from build123d import *

# Parameters (mm, degrees)
SKETCH1_R           = 35
BOSS_EXTRUDE1_DEPTH = 203.105968
SKETCH2_R           = 27.36149988
CUT_EXTRUDE1_DEPTH  = 210.050315085
CHAMFER1_SIZE       = 0.441228


with BuildPart() as part:
    # Sketch1 → Boss-Extrude1 (new body)
    with BuildSketch(Plane(origin=(0, 0, 0), x_dir=(1, 0, 0), z_dir=(0, 1, 0))):
        with Locations(Location((0, 0, 0), (0, 0, 270))):
            Circle(SKETCH1_R)
    extrude(amount=BOSS_EXTRUDE1_DEPTH)

    # Sketch2 → Cut-Extrude1 (cut, through all)
    with BuildSketch(Plane(origin=(0, 0, 0), x_dir=(1, 0, 0), z_dir=(0, 1, 0))):
        with Locations(Location((0, 0, 0), (0, 0, 270))):
            Circle(SKETCH2_R)
    extrude(amount=CUT_EXTRUDE1_DEPTH, mode=Mode.SUBTRACT)

    # Chamfer1
    chamfer1_edges = [part.edges().sort_by_distance(p)[0] for p in [
        (0, 0, -35),
        (0, 203.105968, -35),
        (0, 0, -27.36149988),
        (0, 203.105968, -27.36149988),
    ]]
    chamfer(chamfer1_edges, length=CHAMFER1_SIZE)


solid = part.part
Geometry: final body of the model. Coordinates: model frame, mm. Round coordinates to 2 decimals unless told otherwise and drop trailing zeros. Write each loop counter-clockwise with the first axis right and the second up, starting at its lowest first coordinate (ties: lowest second). Pieces come first, ordered by that corner, then holes. Notation, with made-up numbers: M 61.25,-11 L 95.25,-11 A16 ccw 95.25,4 Z; hole C -9.5,71.25 d8. An arc over 180 degrees is marked long. Write item = value, one per line.
Item 1: Section query C-C on y = 120.5. Return loops of the section in (x, z).
Findings:
outline = C 0,0 d70; hole C 0,0 d54.72
Item 2: Section query B-B on z = 0. Return loops of the section in (x, y), then the cut area to 3 significant figures.
Findings:
outline = M -35,0.44 L -34.56,0 L -27.8,0 L -27.36,0.44 L -27.36,202.66 L -27.8,203.11 L -34.56,203.11 L -35,202.66 Z; M 27.36,0.44 L 27.8,0 L 34.56,0 L 35,0.44 L 35,202.66 L 34.56,203.11 L 27.8,203.11 L 27.36,202.66 Z
area = 3,100 mm^2
Item 3: Section query A-A on x = 0. Return loops of the section in (y, z), then the cut area to 3 significant figures.
Findings:
outline = M 0,-34.56 L 0.44,-35 L 202.66,-35 L 203.11,-34.56 L 203.11,-27.8 L 202.66,-27.36 L 0.44,-27.36 L 0,-27.8 Z; M 0,27.8 L 0.44,27.36 L 202.66,27.36 L 203.11,27.8 L 203.11,34.56 L 202.66,35 L 0.44,35 L 0,34.56 Z
area = 3,100 mm^2
Item 4: Pin query (flat end, axial travel): P1, Ø10, axis at y = 24.5, z = 19.5, coming from the -X side; P2, Ø1, axis at y = 53, z = -13.5, coming from the +X side; P3, Ø3, axis at x = -27, y = 108.5, coming from the -Z side. Return the tip coordinate at first contact, or that it passes through.
Findings:
P1 = -31.86
P2 = 32.5
P3 = -23.97
Item 5: Pull-direction query (Z, two-part tool) for faces 1 (the face through (-21, 100, -28)), 2 (the face through (8.219, 100.137, 26.098)), 3 (the face through (16, 203.106, -23)); classes: pulls with the +Z half, pulls with the -Z half, needs draft (parallel to the pull), parting line crosses it, or undercut.
Findings:
face_1 = parting line crosses it
face_2 = undercut
face_3 = needs draft
Item 6: Material intervals for line 1 along X through (y, z) = (94, 0); line 2 along X through (y, z) = (119, -18.5); line 3 along Z through (x, y) = (-8, 124), sorted ascending. Write a range as [from, to].
Findings:
line_1 = [-35, -27.36], [27.36, 35]
line_2 = [-29.71, -20.16], [20.16, 29.71]
line_3 = [-34.07, -26.17], [26.17, 34.07]
